Part model, mm, in its own coordinate system. Round coordinates to 2 decimals unless told otherwise and drop trailing zeros. Write each loop counter-clockwise with the first axis right and the second up, starting at its lowest first coordinate (ties: lowest second). Pieces come first, ordered by that corner, then holes.
1) Saw through at A-A on x = 30. Write the cut outline in (y, z).
2) Saw through at B-B on y = 0. Write the cut outline in (x, z), and give its area (3 significant figures).
3) Drill centre lines: L1, parallel to Y at x = 30, z = 2.8; L2, parallel to Y at x = -30, z = 1.15; L3, parallel to X at y = -10.25, z = 0.25. Where is each one in solid material? Low to high.
4) Saw through at D-D on x = -30. Write the cut outline in (y, z), and give its area (4 significant figures).
5) Saw through at C-C on z = 1.2. Write the cut outline in (x, y).
```python
from build123d import *

# Parameters (mm, degrees)
ESQUISSE1_R        = 2.25
BOSS_EXTRU_1_DEPTH = 5
TROU_TARAUD_M41_D  = 3.3


with BuildPart() as part:
    # Esquisse1 → Boss.-Extru.1 (new body)
    with BuildSketch(Plane.XY):
        with BuildLine():
            Line((-35, 15), (35, 15))
            ThreePointArc((35, 15), (38.535533906, 13.535533906), (40, 10))
            Line((40, 10), (40, -10))
            ThreePointArc((40, -10), (38.535533906, -13.535533906), (35, -15))
            Line((35, -15), (-35, -15))
            ThreePointArc((-35, -15), (-38.535533906, -13.535533906), (-40, -10))
            Line((-40, -10), (-40, 10))
            ThreePointArc((-40, 10), (-38.535533906, 13.535533906), (-35, 15))
        make_face()
        with Locations((30, 0)):
            Circle(ESQUISSE1_R, mode=Mode.SUBTRACT)
    extrude(amount=BOSS_EXTRU_1_DEPTH)

    # Trou taraudé M41 (through all)
    with Locations(Plane.XY.offset(5)):
        with Locations((-30, 0)):
            Hole(TROU_TARAUD_M41_D / 2)


solid = part.part
```
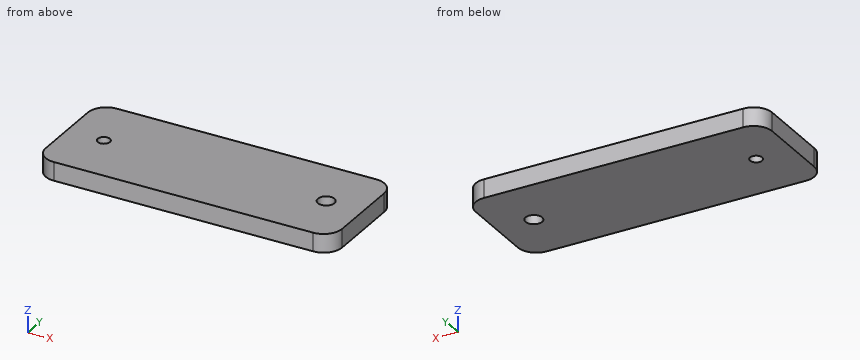
Completed:
1. outline: (-15, 0) - (-2.25, 0) - (-2.25, 5) - (-15, 5) - close; (2.25, 0) - (15, 0) - (15, 5) - (2.25, 5) - close
2. outline: (-40, 0) - (-31.65, 0) - (-31.65, 5) - (-40, 5) - close; (-28.35, 0) - (27.75, 0) - (27.75, 5) - (-28.35, 5) - close; (32.25, 0) - (40, 0) - (40, 5) - (32.25, 5) - close
2. area: 361 mm2
3. L1: y = -15 to -2.25, 2.25 to 15
3. L2: y = -15 to -1.65, 1.65 to 15
3. L3: x = -39.99 to 39.99
4. outline: (-15, 0) - (-1.65, 0) - (-1.65, 5) - (-15, 5) - close; (1.65, 0) - (15, 0) - (15, 5) - (1.65, 5) - close
4. area: 133.5 mm2
5. outline: (-40, -10) arc R5 ccw to (-35, -15) - (35, -15) arc R5 ccw to (40, -10) - (40, 10) arc R5 ccw to (35, 15) - (-35, 15) arc R5 ccw to (-40, 10) - close; hole circle Ø3.3 at (-30, 0); hole circle Ø4.5 at (30, 0)
